```python
from build123d import *

# Parameters (mm, degrees)
SKETCH1_W           = 330.2
SKETCH1_H           = 57.15
BOSS_EXTRUDE1_DEPTH = 6.35
SKETCH3_W           = 24.892
SKETCH3_H           = 12
BOSS_EXTRUDE2_DEPTH = 6.35
SKETCH4_W           = 13.208
SKETCH4_H           = 13.208
CUT_EXTRUDE2_DEPTH  = 171.131311419
SKETCH5_W           = 365.344823274
SKETCH5_H           = 36.987593387
CUT_EXTRUDE3_DEPTH  = 30.796


with BuildPart() as part:
    # Sketch1 → Boss-Extrude1 (new body)
    with BuildSketch(Plane(origin=(0, 0, 0), x_dir=(1, 0, 0), z_dir=(0, 1, 0))):
        Rectangle(SKETCH1_W, SKETCH1_H)
    extrude(amount=BOSS_EXTRUDE1_DEPTH)

    # Sketch3 → Boss-Extrude2 (add)
    with BuildSketch(Plane(origin=(0, 0, 0), x_dir=(1, 0, 0), z_dir=(0, 1, 0))):
        with Locations((-114.3, -34.575)):
            Rectangle(SKETCH3_W, SKETCH3_H)
        with Locations((-76.2, -34.575)):
            Rectangle(SKETCH3_W, SKETCH3_H)
        with Locations((-38.1, -34.575)):
            Rectangle(SKETCH3_W, SKETCH3_H)
        with Locations((0, -34.575)):
            Rectangle(SKETCH3_W, SKETCH3_H)
        with Locations((38.1, -34.575)):
            Rectangle(SKETCH3_W, SKETCH3_H)
        with Locations((76.2, -34.575)):
            Rectangle(SKETCH3_W, SKETCH3_H)
        with Locations((114.3, -34.575)):
            Rectangle(SKETCH3_W, SKETCH3_H)
        with Locations((152.4, -34.575)):
            Rectangle(SKETCH3_W, SKETCH3_H)
        with Locations((-152.4, -34.575)):
            Rectangle(SKETCH3_W, SKETCH3_H)
    extrude(amount=BOSS_EXTRUDE2_DEPTH)

    # Sketch4 → Cut-Extrude2 (cut, through all)
    with BuildSketch(Plane(origin=(0, 0, 0), x_dir=(1, 0, 0), z_dir=(0, 1, 0))):
        with Locations((165.1, 16.575)):
            Rectangle(SKETCH4_W, SKETCH4_H)
        with Locations((-165.1, -34.225)):
            Rectangle(SKETCH4_W, SKETCH4_H)
        with Locations((165.1, -8.825)):
            Rectangle(SKETCH4_W, SKETCH4_H)
        with Locations((165.1, -34.225)):
            Rectangle(SKETCH4_W, SKETCH4_H)
        with Locations((-165.1, -8.825)):
            Rectangle(SKETCH4_W, SKETCH4_H)
        with Locations((-165.1, 16.575)):
            Rectangle(SKETCH4_W, SKETCH4_H)
    extrude(amount=CUT_EXTRUDE2_DEPTH, mode=Mode.SUBTRACT)

    # Sketch5 → Cut-Extrude3 (cut)
    with BuildSketch(Plane(origin=(0, 0, -28.575), x_dir=(-1, 0, 0), z_dir=(0, 0, -1))):
        with Locations((-4.838573854, 1.285089719)):
            Rectangle(SKETCH5_W, SKETCH5_H)
    extrude(amount=-CUT_EXTRUDE3_DEPTH, mode=Mode.SUBTRACT)


solid = part.part
```
Could you check a few things on this model? Use its own coordinates, in mm. A direction names the side the tool comes from. Coordinates: 2 decimals unless noted, no trailing zeros. Order: outer loops, then holes, each group sorted by start corner. A loop starts at its lowest first (then second) coordinate and runs counter-clockwise, first axis right, second up. Notation, with made-up numbers: M 43,41 L 87,41 A19 cw 87,47 Z; hole C 68.5,-34 d6. An arc over 180 degrees is marked long. Use a Markdown table: item, result. Add a question column.
Q1. We'd pull the mould along X, two halves only. Please class faces 1 (the flat face through (-114, 3, 40.575)), 2 (the flat face through (165.1, 3, 22)), 3 (the flat face through (-25.654, 3, 35)), 4 (the flat face through (-158.496, 3, 9)): pulls with the +X half, pulls with the -X half, needs draft (parallel to the pull), parting line crosses it, or undercut.
Q2. I'm going to push flat-ended pins straight in: pin 1 (3 mm diameter, centred on x = -20.5, y = 4, fed in from +Z) (3 decimals); pin 2 (1.9 mm diameter, centred on y = 2.5, z = 33.5, fed in from -X); pin 3 (3 mm diameter, centred on y = 2.5, z = 37.5, fed in from +X). Where does each tip first touch, or does it pass through?
Q3. I want a section at B-B on x = -132.5. List the corners of the cut face in (y, z) for me (3 decimals).
Q4. If I drill on L1, parallel to X at y = 4.5, z = 5; L2, parallel to Z at x = 101, y = 4 (3 decimals), over which ranges is the centre line in solid material (lowest first)?
Q5. Which directions (+Z, -Z, +X, -X, +Y, -Y) give clear straight access to the entire face, cutting with the end or side of a thin tool? Please do faces 5 (the flat face through (-12.446, 3, 35)), 6 (the flat face through (158.496, 3, 9)), 7 (the flat face through (-162, 3, 27.621)).
Q6. I want a section at A-A on z = 12. List the corners of the cut face in (x, y) for me, then the cut area to 3 significant figures.
Checked values:
| question | item | result |
|---|---|---|
| 1 | face 1 | needs draft |
| 1 | face 2 | pulls with the +X half |
| 1 | face 3 | undercut |
| 1 | face 4 | pulls with the -X half |
| 2 | pin 1 | z = 28.575 |
| 2 | pin 2 | x = -158.5 |
| 2 | pin 3 | x = 158.5 |
| 3 | outline | M 0,2.221 L 6.35,2.221 L 6.35,28.575 L 0,28.575 Z |
| 4 | L1 | -158.5 to 158.5 |
| 4 | L2 | 2.221 to 28.575 |
| 5 | face 5 | +Z, +Y, -Y |
| 5 | face 6 | -Z, +X, +Y, -Y |
| 5 | face 7 | +Z, -X, +Y, -Y |
| 6 | outline | M -158.5,0 L 158.5,0 L 158.5,6.35 L -158.5,6.35 Z |
| 6 | area | 2,010 mm² |
